```python
from build123d import *

# Parameters (mm, degrees)
SKETCH_1_R      = 17.5
SKETCH_1_R_2    = 1
EXTRUDE_1_DEPTH = 2


with BuildPart() as part:
    # Эскиз1 → Бобышка-Вытянуть1 (new body)
    with BuildSketch(Plane.XY):
        Circle(SKETCH_1_R)
        with Locations((0, 10)):
            Circle(SKETCH_1_R_2, mode=Mode.SUBTRACT)
        with Locations((0, -10)):
            Circle(SKETCH_1_R_2, mode=Mode.SUBTRACT)
        with BuildLine():
            Line((2.681883666, 2.9), (-2.681883666, 2.9))
            ThreePointArc((-2.681883666, 2.9), (0, -3.95), (2.681883666, 2.9))
        make_face(mode=Mode.SUBTRACT)
    extrude(amount=EXTRUDE_1_DEPTH)


solid = part.part
```
Design review of the part built by this model. Coordinates are the model's own, in mm. A direction names the side the tool comes from. Give positions to 0.01 mm unless a question says otherwise; leave off trailing zeros. Write each loop counter-clockwise with the first axis right and the second up, starting at its lowest first coordinate (ties: lowest second). Pieces come first, ordered by that corner, then holes. Notation, with made-up numbers: (82, -2.75) - (132, -2.75) arc R17 ccw to (132, 12.25) - close; hole circle Ø2 at (16.25, 48.5). An arc over 180 degrees is marked (long way). Return JSON: item names as keys, results as strings. Group by question number.
(1) To check wall thickness, follow probe 1 along X at (y, z) = (0.5, 1.25); probe 2 along X at (y, z) = (11.5, 1); probe 3 along Y at (x, z) = (-4, 0.4). State the ranges of each line that lie inside material, in increasing order.
(2) Insertion check: pin 1 (6.5 mm diameter, centred on x = 0, y = 0, fed in from +Z). The pin has a flat end and moves straight along its axis. Give the tip position at first contact, or say it passes through.
(3) Mouldability with a two-part tool opening along X and no side actions: class faces 1 (the flat face through (-4.1, 0.2, 2)), 2 (the cylindrical face through (-13.887, -10.648, 0.986)), 3 (the cylindrical face through (0, 11, 1)) as +X half, -X half, draft (parallel to the pull), parting line (faces both ways), or undercut.
(4) We need section D-D, the plane y = -10. Give the boundary of the cut face in (x, z), then the cut area to 3 significant figures.
(5) Machinability: for faces 4 (the flat face through (-4.1, 0.2, 0)), 5 (the flat face through (0, 2.9, 1)), which of the approach directions +Z, -Z, +X, -X, +Y, -Y give a long, thin tool a straight path to every point of the face, cutting with its end or side? Answer none if there is none.
(6) We need section A-A, the plane y = 0. Give the boundary of the cut face in (x, z).
(7) We need section B-B, the plane x = 0. Give the boundary of the cut face in (y, z), then the cut area to 3 significant figures.
(8) We need section C-C, the plane z = 1.4. Give the boundary of the cut face in (x, y), then the cut area to 3 significant figures.
Reported:
{
 "1": {"probe 1": "x = -17.49 to -3.92, 3.92 to 17.49", "probe 2": "x = -13.19 to 13.19", "probe 3": "y = -17.04 to 17.04"},
 "2": {"pin 1": "stops at z = 2"},
 "3": {"face 1": "draft", "face 2": "parting line", "face 3": "undercut"},
 "4": {"outline": "(-14.36, 0) - (-1, 0) - (-1, 2) - (-14.36, 2) - close; (1, 0) - (14.36, 0) - (14.36, 2) - (1, 2) - close", "area": "53.4 mm2"},
 "5": {"face 4": "-Z, +X, -X, +Y, -Y", "face 5": "+Z, -Z"},
 "6": {"outline": "(-17.5, 0) - (-3.95, 0) - (-3.95, 2) - (-17.5, 2) - close; (3.95, 0) - (17.5, 0) - (17.5, 2) - (3.95, 2) - close"},
 "7": {"outline": "(-17.5, 0) - (-11, 0) - (-11, 2) - (-17.5, 2) - close; (-9, 0) - (-3.95, 0) - (-3.95, 2) - (-9, 2) - close; (2.9, 0) - (9, 0) - (9, 2) - (2.9, 2) - close; (11, 0) - (17.5, 0) - (17.5, 2) - (11, 2) - close", "area": "48.3 mm2"},
 "8": {"outline": "circle Ø35 at (0, 0); hole (-2.68, 2.9) arc R3.95 ccw (long way) to (2.68, 2.9) - close; hole circle Ø2 at (0, -10); hole circle Ø2 at (0, 10)", "area": "911 mm2"}
}
